from build123d import *

# Parameters (mm, degrees)
SKETCH2_W           = 150
SKETCH2_H           = 90
BOSS_EXTRUDE1_DEPTH = 3
SKETCH3_W           = 60
SKETCH3_H           = 90
BOSS_EXTRUDE2_DEPTH = 10
SKETCH4_W           = 40
SKETCH4_H           = 20
BOSS_EXTRUDE3_DEPTH = 40


with BuildPart() as part:
    # Sketch2 → Boss-Extrude1 (new body)
    with BuildSketch(Plane(origin=(0, 0, 0), x_dir=(0, 1, 0), z_dir=(0, 0, 1))):
        with Locations((75, 45)):
            Rectangle(SKETCH2_W, SKETCH2_H)
    extrude(amount=BOSS_EXTRUDE1_DEPTH)

    # Sketch3 → Boss-Extrude2 (add)
    with BuildSketch(Plane.XY.offset(3)):
        with Locations((-45, 60)):
            Rectangle(SKETCH3_W, SKETCH3_H)
    extrude(amount=BOSS_EXTRUDE2_DEPTH)

    # Sketch4 → Boss-Extrude3 (add)
    with BuildSketch(Plane.XY.offset(3)):
        with Locations((-45, 130)):
            Rectangle(SKETCH4_W, SKETCH4_H)
    extrude(amount=BOSS_EXTRUDE3_DEPTH)


solid = part.part
Can you work these out from the model? Positions are in its coordinate system, mm. A direction names the side the tool comes from. Coordinates: 2 decimals unless noted, no trailing zeros. Order: outer loops, then holes, each group sorted by start corner. A loop starts at its lowest first (then second) coordinate and runs counter-clockwise, first axis right, second up. Notation, with made-up numbers: (76, 17) - (95, 17) arc R25 cw to (95, 35) - close; hole circle Ø1 at (46.5, 5.5). An arc over 180 degrees is marked (long way). Answer as a JSON object with one key per item and string values. Group by question number.
Q1. Will these pins go through, and if not, where does the flat tip stop? P1, Ø8, axis at y = 74.5, z = 9.5, coming from the -X side; P2, Ø12, axis at x = -19, z = 9.5, coming from the -Y side; P3, Ø16, axis at y = 128.5, z = 30.5, coming from the -X side.
Q2. Imagine slicing it at B-B (x = -70). Please give me the cut outline in (y, z).
Q3. Imagine slicing it at D-D (x = -45). Please give me the cut outline in (y, z), and give its area (3 significant figures).
Q4. We'd pull the mould along Y, two halves only. Please class faces 1 (the face through (-44, 0, 1)), 2 (the face through (-45, 140, 23)), 3 (the face through (-15, 59, 8)), 4 (the face through (-45, 120, 23)): +Y half, -Y half, draft (parallel to the pull), parting line (faces both ways), or undercut.
Q5. On a 3-axis mill with a long thin cutter (end or side, diameter ignored), from which of +Z, -Z, +X, -X, +Y, -Y can I reach the whole of each face in a straight line? I mean faces 5 (the face through (-45, 61, 13)), 6 (the face through (-25, 130, 23)), 7 (the face through (-45, 105, 8)). Say none if no direction works.
Q6. I need wall thicknesses on line 1 (Y direction, x = -34, z = 12.5); line 2 (Z direction, x = -26, y = 61.5); line 3 (X direction, y = 20.5, z = 7). Which ranges of each line are inside material? Lowest first, please. Write a range as from..to.
Q7. Imagine slicing it at C-C (z = 36.5). Please give me the cut outline in (x, y), and give its area (3 significant figures).
Q8. Imagine slicing it at A-A (y = 89.5). Please give me the cut outline in (x, z), and give its area (3 significant figures).
Determined:
{
 "1": {"P1": "stops at x = -75", "P2": "stops at y = 15", "P3": "stops at x = -65"},
 "2": {"outline": "(0, 0) - (150, 0) - (150, 3) - (105, 3) - (105, 13) - (15, 13) - (15, 3) - (0, 3) - close"},
 "3": {"outline": "(0, 0) - (150, 0) - (150, 3) - (140, 3) - (140, 43) - (120, 43) - (120, 3) - (105, 3) - (105, 13) - (15, 13) - (15, 3) - (0, 3) - close", "area": "2,150 mm2"},
 "4": {"face 1": "-Y half", "face 2": "+Y half", "face 3": "draft", "face 4": "undercut"},
 "5": {"face 5": "+Z, +X, -X, -Y", "face 6": "+Z, +X, +Y", "face 7": "+Z, +X, -X"},
 "6": {"line 1": "y = 15..105, 120..140", "line 2": "z = 0..13", "line 3": "x = -75..-15"},
 "7": {"outline": "(-65, 120) - (-25, 120) - (-25, 140) - (-65, 140) - close", "area": "800 mm2"},
 "8": {"outline": "(-90, 0) - (0, 0) - (0, 3) - (-15, 3) - (-15, 13) - (-75, 13) - (-75, 3) - (-90, 3) - close", "area": "870 mm2"}
}
